```python
from build123d import *

# Parameters (mm, degrees)
F1_DEPTH = 25.4
F2_W     = 25.4
F2_H     = 12.7
F3_DEPTH = 25.4
F4_R     = 3.175
F5_DEPTH = 12.7


with BuildPart() as f1:
    # F0 (on Top) → F1 (new body)
    with BuildSketch(Plane.XY):
        Polygon((76.2, 0), (0, 0), (38.1, -25.4), (76.2, -25.4), align=None)
    extrude(amount=F1_DEPTH)

    # F2 (on face) → F3 (cut)
    with BuildSketch(Plane.XY.offset(25.4)):
        with Locations((57.15, -19.05)):
            Rectangle(F2_W, F2_H)
    extrude(amount=-F3_DEPTH, mode=Mode.SUBTRACT)

    # F4 (on face) → F5 (cut)
    with BuildSketch(Plane.XZ.offset(12.7)):
        with Locations((57.15, 12.7)):
            Circle(F4_R)
    extrude(amount=-F5_DEPTH, mode=Mode.SUBTRACT)

    # F6: F1 across plane


with BuildPart() as f1_1:
    add(f1.part)
    add(f1.part.mirror(Plane.XZ))


solid = f1_1.part
```
Here's how the part is built. I have some questions about the finished solid (model axes, mm). A direction names the side the tool comes from. Give positions to 0.01 mm unless a question says otherwise; leave off trailing zeros. Loops run counter-clockwise (first coordinate to the right, second up) from the corner with the lowest first, then second, coordinate; pieces in that order, holes last. Notation, with made-up numbers: (21.5, 56.5) -> (38.5, 56.5) arc R6 ccw to (38.5, 62.5) -> close; hole circle Ø9 at (-7.75, 53.25). An arc over 180 degrees is marked (long way). Use one line per item in the form item = value. Start each with the question number.
1) Imagine slicing it at B-B (z = 12.7). Please give me the cut outline in (x, y) (3 decimals).
2) For P1, Ø4, axis at x = 57.15, z = 12.7, coming from the -Y side; P2, Ø7.5, axis at x = 59.5, z = 11.5, coming from the +Y side; P3, Ø5, axis at y = 17.5, z = 11, coming from the -X side; P4, Ø6.5, axis at y = -18.5, z = 16, coming from the -X side (3 decimals), each with a flat end and sliding along its axis, tell me the tip position at first contact or that it passes through.
3) Which directions (+Z, -Z, +X, -X, +Y, -Y) give clear straight access to the entire face, cutting with the end or side of a thin tool? Please do faces 4 (the face through (54, 12.7, 10)), 5 (the face through (46, 0, 0)), 6 (the face through (69.85, -19, 13)).
4) Imagine slicing it at D-D (y = 11). Please give me the cut outline in (x, z) (3 decimals), then the cut area to 3 significant figures.
5) Thinking about a two-plate mould opening in X: for faces 1 (the face through (73, -25.4, 13)), 2 (the face through (69.85, 19, 13)), 3 (the face through (18.78, 12.52, 12.52)), which applies, +X half, -X half, draft (parallel to the pull), parting line (faces both ways), or undercut?
6) Imagine slicing it at C-C (x = 57.15). Please give me the cut outline in (y, z) (3 decimals).
7) Please list where these lines run through material, in increasing order: line 1 along Z through (x, y) = (57.15, -3.25) (3 decimals); line 2 along Y through (x, z) = (61, 10); line 3 along Z through (x, y) = (55, 2).
8) Imagine slicing it at A-A (y = 19.5). Please give me the cut outline in (x, z), then the cut area to 3 significant figures.
Check values:
q1.outline = (0, 0) -> (38.1, -25.4) -> (44.45, -25.4) -> (44.45, -12.7) -> (53.975, -12.7) -> (53.975, 12.7) -> (44.45, 12.7) -> (44.45, 25.4) -> (38.1, 25.4) -> close; (60.325, -12.7) -> (69.85, -12.7) -> (69.85, -25.4) -> (76.2, -25.4) -> (76.2, 25.4) -> (69.85, 25.4) -> (69.85, 12.7) -> (60.325, 12.7) -> close
q2.P1 = through
q2.P2 = 12.7
q2.P3 = 22.5
q2.P4 = 22.875
q3.face_4 = +Z, -Z, +Y
q3.face_5 = -Z, +X, -X, +Y, -Y
q3.face_6 = +Z, -Z, -Y
q4.outline = (16.5, 0) -> (76.2, 0) -> (76.2, 25.4) -> (16.5, 25.4) -> close; hole circle Ø6.35 at (57.15, 12.7)
q4.area = 1,480 mm^2
q5.face_1 = draft
q5.face_2 = undercut
q5.face_3 = -X half
q6.outline = (-12.7, 0) -> (12.7, 0) -> (12.7, 9.525) -> (-12.7, 9.525) -> close; (-12.7, 15.875) -> (12.7, 15.875) -> (12.7, 25.4) -> (-12.7, 25.4) -> close
q7.line_1 = 0 to 9.525, 15.875 to 25.4
q7.line_2 = -12.7 to 12.7
q7.line_3 = 0 to 10.36, 15.04 to 25.4
q8.outline = (29.25, 0) -> (44.45, 0) -> (44.45, 25.4) -> (29.25, 25.4) -> close; (69.85, 0) -> (76.2, 0) -> (76.2, 25.4) -> (69.85, 25.4) -> close
q8.area = 547 mm^2
